Check sheet for the modelled part. Datum: model origin and axes. Units: mm. A direction names the side the tool comes from. Round coordinates to 2 decimals unless told otherwise and drop trailing zeros. Order: outer loops, then holes, each group sorted by start corner. A loop starts at its lowest first (then second) coordinate and runs counter-clockwise, first axis right, second up.
(1) Depth check by flat-ended pin: pin 1 (9 mm diameter, centred on x = -34, z = -19, fed in from +Y); pin 2 (4 mm diameter, centred on x = 34, z = -19, fed in from +Y); pin 3 (5 mm diameter, centred on x = -22, y = 30.5, fed in from -Z). Enter the tip coordinate at first touch or a pass-through.
(2) Sectioned sample at B-B, the plane z = 19. Count the separate pieces of the cut face and the enclosed holes in it, and give its area (3 significant figures).
(3) Thickness scan on probe 1 along Z at (x, y) = (34, 11); probe 2 along Z at (x, y) = (-38, 38.5); probe 3 along X at (y, z) = (41.2, -19). Record the ranges inside material, lowest first.
(4) Sectioned sample at C-C, the plane x = 2. Enter the section's corners in (y, z), and give its area (3 significant figures).
(5) Sectioned sample at A-A, the plane z = 8. Enter the section's corners in (x, y).
(6) Tool access check on faces 1 (the flat face through (25.25, 38, -19)), 2 (the flat face through (40, 27, 0)), 3 (the flat face through (-36, 37, 24.25)). Record the directions out of +Z, -Z, +X, -X, +Y, -Y that give a thin tool (end or side, any length) a straight path to the whole face; none if there is none.
```python
from build123d import *

# Parameters (mm, degrees)
BOSS_EXTRUDE1_DEPTH  = 36
M3_CLEARANCE_HOLE1_D = 4
SKETCH6_W            = 94.5
SKETCH6_H            = 86
SKETCH6_W_2          = 27
SKETCH6_H_2          = 27
BOSS_EXTRUDE2_DEPTH  = 8.7
FILLET1_R            = 2.5
SKETCH2_3_W          = 3.25
SKETCH2_3_H          = 6.25
CUT_EXTRUDE1_DEPTH   = 27
CUT_EXTRUDE2_DEPTH   = 108.826956277
M6_CLEARANCE_HOLE1_D = 7
SKETCH12_W           = 10.5
SKETCH12_H           = 5.25
CUT_EXTRUDE4_DEPTH   = 22


with BuildPart() as part:
    # Sketch2 → Boss-Extrude1 (new body)
    with BuildSketch(Plane(origin=(0, 0, 0), x_dir=(1, 0, 0), z_dir=(0, 1, 0))):
        Polygon((-33.75, 13), (-26, 13), (-26, 43), (-47.25, 43), (-47.25, -43), (47.25, -43), (47.25, 43), (26, 43), (26, 13), (33.75, 13), (33.75, -13), (15.75, -13), (15.75, -15), (-15.75, -15), (-15.75, -13), (-33.75, -13), align=None)
    extrude(amount=BOSS_EXTRUDE1_DEPTH)

    # M3 Clearance Hole1 (through all)
    with Locations(Plane(origin=(47.25, 0, 0), x_dir=(0, 0, -1), z_dir=(1, 0, 0))):
        with Locations((0, 24)):
            Hole(M3_CLEARANCE_HOLE1_D / 2)

    # Sketch6 → Boss-Extrude2 (add)
    with BuildSketch(Plane(origin=(0, 36, 0), x_dir=(1, 0, 0), z_dir=(0, 1, 0))):
        Rectangle(SKETCH6_W, SKETCH6_H)
        Rectangle(SKETCH6_W_2, SKETCH6_H_2, mode=Mode.SUBTRACT)
    extrude(amount=BOSS_EXTRUDE2_DEPTH)

    # Fillet1
    fillet1_edges = [part.edges().sort_by_distance(p)[0] for p in [
        (47.25, 22.35, -43),
        (47.25, 22.35, 43),
        (-47.25, 22.35, 43),
        (-47.25, 22.35, -43),
    ]]
    fillet(fillet1_edges, radius=FILLET1_R)

    # Sketch2<3> → Cut-Extrude1 (cut)
    with BuildSketch(Plane(origin=(0, 0, 0), x_dir=(1, 0, 0), z_dir=(0, 1, 0))):
        with Locations((-40.5, 0)):
            Rectangle(SKETCH2_3_W, SKETCH2_3_H)
        with Locations((40.5, 0)):
            Rectangle(SKETCH2_3_W, SKETCH2_3_H)
    extrude(amount=CUT_EXTRUDE1_DEPTH, mode=Mode.SUBTRACT)

    # Sketch8 → Cut-Extrude2 (cut, through all)
    with BuildSketch(Plane.XY.offset(43)):
        with BuildLine():
            Line((-8, 22), (-8, 0))
            Line((-8, 0), (8, 0))
            Line((8, 0), (8, 22))
            ThreePointArc((8, 22), (0, 30), (-8, 22))
        make_face()
    extrude(amount=-CUT_EXTRUDE2_DEPTH, mode=Mode.SUBTRACT)

    # M6 Clearance Hole1 (through all)
    with Locations(Plane(origin=(0, 44.7, 0), x_dir=(1, 0, 0), z_dir=(0, 1, 0))):
        with Locations((-34, 19), (34, 19), (34, -19), (-34, -19)):
            Hole(M6_CLEARANCE_HOLE1_D / 2)

    # Sketch12 → Cut-Extrude4 (cut)
    with BuildSketch(Plane(origin=(47.25, 0, 0), x_dir=(0, 0, -1), z_dir=(1, 0, 0))):
        with Locations((-19, 37.075)):
            Rectangle(SKETCH12_W, SKETCH12_H)
        with Locations((19, 37.075)):
            Rectangle(SKETCH12_W, SKETCH12_H)
    cut_extrude4 = extrude(amount=-CUT_EXTRUDE4_DEPTH, mode=Mode.SUBTRACT)

    # Mirror2: Cut-Extrude4 across plane
    add(cut_extrude4.mirror(Plane(origin=(0, 0, 0), x_dir=(0, 0, 1), z_dir=(1, 0, 0))), mode=Mode.SUBTRACT)


solid = part.part
```
Derived:
1. pin 1: stops at y = 44.7
1. pin 2: passes through
1. pin 3: stops at z = 13
2. separate pieces: 5
2. enclosed holes: 0
2. area: 2,990 mm2
3. probe 1: z = -43 to -22.5, -15.5 to 15.5, 22.5 to 43
3. probe 2: z = -43 to -24.25, -13.75 to 13.75, 24.25 to 43
3. probe 3: x = -47.25 to -37.5, -30.5 to 30.5, 37.5 to 47.25
4. outline: (29.75, 15) - (36, 15) - (36, 13.5) - (44.7, 13.5) - (44.7, 43) - (29.75, 43) - close; (36, -43) - (44.7, -43) - (44.7, -13.5) - (36, -13.5) - close
4. area: 688 mm2
5. outline: (-47.25, 0) - (-33.75, 0) - (-33.75, 36) - (-13.5, 36) - (-13.5, 44.7) - (-47.25, 44.7) - close; (13.5, 36) - (33.75, 36) - (33.75, 0) - (47.25, 0) - (47.25, 44.7) - (13.5, 44.7) - close
6. face 1: +X, -Y
6. face 2: -Y
6. face 3: -X
